Source: CAD feature listing. Evaluate the final solid. Frame: model axes, mm. Coordinates: 2 decimals unless noted, no trailing zeros. Loops run counter-clockwise (first coordinate to the right, second up) from the corner with the lowest first, then second, coordinate; pieces in that order, holes last.
from build123d import *

# Parameters (mm, degrees)
SKETCH1_W                      = 98
SKETCH1_H                      = 98
BOSS_EXTRUDE1_DEPTH            = 1.5
SKETCH2_W                      = 10
SKETCH2_H                      = 10
CUT_EXTRUDE1_DEPTH             = 10
F_3_0_3_DIAMETER_HOLE1_D       = 3
SKETCH5_W                      = 25
SKETCH5_H                      = 13
CUT_EXTRUDE2_DEPTH             = 10
F_2_3_2_3_DIAMETER_HOLE1_D     = 2.3
F_2_3_2_3_DIAMETER_HOLE1_DEPTH = 30
SKETCH8_R                      = 1.5
CUT_EXTRUDE3_DEPTH             = 10
F_3_0_3_DIAMETER_HOLE2_D       = 3
F_3_0_3_DIAMETER_HOLE2_DEPTH   = 6.5


with BuildPart() as part:
    # Sketch1 → Boss-Extrude1 (new body)
    with BuildSketch(Plane.XY):
        Rectangle(SKETCH1_W, SKETCH1_H)
    extrude(amount=BOSS_EXTRUDE1_DEPTH)

    # Sketch2 → Cut-Extrude1 (cut)
    with BuildSketch(Plane.XY.offset(1.5)):
        with Locations((-44, 44)):
            Rectangle(SKETCH2_W, SKETCH2_H)
        with Locations((44, 44)):
            Rectangle(SKETCH2_W, SKETCH2_H)
        with Locations((44, -44)):
            Rectangle(SKETCH2_W, SKETCH2_H)
        with Locations((-44, -44)):
            Rectangle(SKETCH2_W, SKETCH2_H)
    extrude(amount=-CUT_EXTRUDE1_DEPTH, mode=Mode.SUBTRACT)

    # Ø3.0 (3) Diameter Hole1 (through all)
    with Locations(Plane(origin=(0, 0, 0), x_dir=(-1, 0, 0), z_dir=(0, 0, -1))):
        with Locations((-23, 45.5), (23, 45.5), (45.5, 23), (45.5, -23), (23, -45.5), (-23, -45.5), (-45.5, -23), (-45.5, 23)):
            Hole(F_3_0_3_DIAMETER_HOLE1_D / 2)

    # Sketch5 → Cut-Extrude2 (cut)
    with BuildSketch(Plane.XY.offset(1.5)):
        with Locations((-25.5, 0)):
            Rectangle(SKETCH5_W, SKETCH5_H)
        with Locations((25.5, 0)):
            Rectangle(SKETCH5_W, SKETCH5_H)
    extrude(amount=-CUT_EXTRUDE2_DEPTH, mode=Mode.SUBTRACT)

    # Ø2.3 (2.3) Diameter Hole1
    with Locations(Plane.XY.offset(1.5)):
        with Locations((-22.24500144, -31.590736692), (-22.203117232, 32.633806534), (22.203117232, 32.633806534), (22.24500144, -31.590736692)):
            Hole(F_2_3_2_3_DIAMETER_HOLE1_D / 2, depth=F_2_3_2_3_DIAMETER_HOLE1_DEPTH)

    # Sketch8 → Cut-Extrude3 (cut)
    with BuildSketch(Plane(origin=(0, 0, 0), x_dir=(-1, 0, 0), z_dir=(0, 0, -1))):
        with Locations((-5.7, -0.8)):
            Circle(SKETCH8_R)
    extrude(amount=-CUT_EXTRUDE3_DEPTH, mode=Mode.SUBTRACT)

    # Ø3.0 (3) Diameter Hole2
    with Locations(Plane(origin=(0, 0, 0), x_dir=(-1, 0, 0), z_dir=(0, 0, -1))):
        with Locations((-1.4, -5.5), (-8.2, -5.5)):
            Hole(F_3_0_3_DIAMETER_HOLE2_D / 2, depth=F_3_0_3_DIAMETER_HOLE2_DEPTH)


solid = part.part
Q1. Section C-C, the plane x = -31. Return the cut outline in (y, z).
Q2. Section B-B, the plane y = -0.8. Return the cut outline in (x, z), plus the area to 3 significant figures.
Q3. Contact query for flat-ended pins moving along their axis: pin 1 Ø3 at (x, y) = (6, 27.5) entering from -Z; pin 2 Ø0.8 at (y, z) = (-46, 0.5) entering from -X; pin 3 Ø0.8 at (x, z) = (46, 1) entering from +Y. Output: stop coordinate, or through.
Q4. Line query: line 1 along Y through (x, z) = (45.5, 0.95); line 2 along Y through (x, z) = (-15, 0.5); line 3 along X through (y, z) = (32, 0.5). Output: solid intervals per line, ascending.
Q5. Section A-A, the plane y = 45.5. Return the cut outline in (x, z).
Q6. Draft query along Y for faces 1 (the cylindrical face through (-47, -23, 1)), 2 (the flat face through (-1, 1, 0)). Return one class per face: +Y half, -Y half, draft (parallel to the pull), parting line (faces both ways), or undercut.
Q7. Section D-D, the plane y = 23. Return the cut outline in (x, z), plus the area to 3 significant figures.
Derived:
1. outline: (-49, 0) - (-6.5, 0) - (-6.5, 1.5) - (-49, 1.5) - close; (6.5, 0) - (49, 0) - (49, 1.5) - (6.5, 1.5) - close
2. outline: (-49, 0) - (-38, 0) - (-38, 1.5) - (-49, 1.5) - close; (-13, 0) - (4.2, 0) - (4.2, 1.5) - (-13, 1.5) - close; (7.2, 0) - (13, 0) - (13, 1.5) - (7.2, 1.5) - close; (38, 0) - (49, 0) - (49, 1.5) - (38, 1.5) - close
2. area: 67.5 mm2
3. pin 1: stops at z = 0
3. pin 2: stops at x = -39
3. pin 3: stops at y = 39
4. line 1: y = -39 to -24.5, -21.5 to 21.5, 24.5 to 39
4. line 2: y = -49 to -6.5, 6.5 to 49
4. line 3: x = -49 to -23.16, -21.24 to 21.24, 23.16 to 49
5. outline: (-39, 0) - (-24.5, 0) - (-24.5, 1.5) - (-39, 1.5) - close; (-21.5, 0) - (21.5, 0) - (21.5, 1.5) - (-21.5, 1.5) - close; (24.5, 0) - (39, 0) - (39, 1.5) - (24.5, 1.5) - close
6. face 1: undercut
6. face 2: draft
7. outline: (-49, 0) - (-47, 0) - (-47, 1.5) - (-49, 1.5) - close; (-44, 0) - (44, 0) - (44, 1.5) - (-44, 1.5) - close; (47, 0) - (49, 0) - (49, 1.5) - (47, 1.5) - close
7. area: 138 mm2
